Build history of the part. All positions in model axes, mm. Face numbers are marked on the shaded views. A direction names the side the tool comes from. Coordinates: 2 decimals unless noted, no trailing zeros. Loops run counter-clockwise (first coordinate to the right, second up) from the corner with the lowest first, then second, coordinate; pieces in that order, holes last.
Item 1: Cut at A-A (y = 2.5). Count the separate pieces of the cut face and the enclosed holes in it, and give its area (3 significant figures).
Item 2: Cut at B-B (x = 2.5). List the corners of the cut face in (y, z) (3 decimals).
Item 3: Mould opens along X. For the marked faces 1, 2, 3 and 4 say: released by +X, released by -X, zero draft, split by the parting line, or undercut.
Item 4: 3-axis set-ups, long thin cutter, end or side, ignore diameter. For the marked faces 5, 6 and 7: which of +Z, -Z, +X, -X, +Y, -Y reach the whole face in a straight line?
Item 5: Drill centre lines: line 1 along X through (y, z) = (6.25, -0.9); line 2 along X through (y, z) = (6.5, 0.3) (3 decimals); line 3 along X through (y, z) = (5.5, -0.1). Where is each one in solid material? Low to high.
Item 6: Flat gauge pins, fed straight in: pin 1 (2 mm diameter, centred on x = 3.5, z = 2.5, fed in from +Y); pin 2 (0.8 mm diameter, centred on x = -3, z = -2, fed in from -Y). Where does each tip first touch, or does it go through?
Item 7: Cut at D-D (y = 4.75). List the corners of the cut face in (x, z), and give its area (3 significant figures).
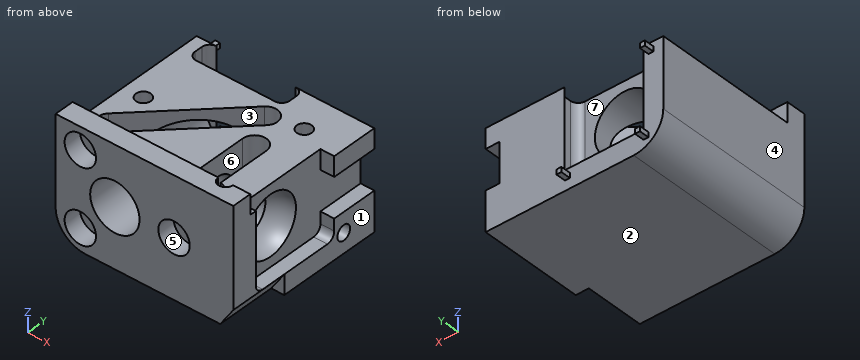
from build123d import *

# Parameters (mm, degrees)
SKETCH1_W                       = 9
SKETCH1_H                       = 6
MAIN_BODY_EXT_DEPTH             = 8.3
EMISSION_PATH_EXT_DEPTH         = 9
SKETCH3_R                       = 1.25
EMISSION_AND_GRIN_CUT_DEPTH     = 19.125672401
SKETCH4_R                       = 1
DRUM_LENS_CUT_DEPTH             = 7
SKETCH5_W                       = 9
SKETCH5_H                       = 7.3
FILTERSET_CUT1_DEPTH            = 1
FILTERSET_CUT2_DEPTH            = 4
SKETCH10_R                      = 2.5
EMISSION_LENS_CUT_DEPTH         = 8.5
SKETCH15_R                      = 0.795
MAGNETS_CUT_DEPTH               = 0.9
SCREW_HOLES_CUT_DEPTH           = 19.561788707
SCREW_HOLES_CUT_DEPTH_BACK      = 3
SKETCH18_R                      = 0.375
EXTERNAL_FILLET_1_R             = 1.5
CUT_EXTRUDE8_DEPTH              = 12.545128843
CUT_EXTRUDE8_DEPTH_BACK         = 4
SKETCH28_R                      = 1.5
CUT_EXTRUDE9_DEPTH              = 3
CUT_EXTRUDE10_DEPTH             = 0.7
SKETCH29_R                      = 0.375
CUT_EXTRUDE11_DEPTH             = 2.5
SKETCH32_W                      = 2
SKETCH32_H                      = 2.36
CUT_EXTRUDE14_DEPTH             = 0.7
CUT_EXTRUDE16_DEPTH             = 9
CUT_EXTRUDE17_REACH             = 12.329
SKETCH37_R                      = 2
CUT_EXTRUDE18_START             = -9
CUT_EXTRUDE18_DEPTH             = 9
CUT_EXTRUDE19_REACH             = 20.126
SKETCH39_W                      = 5.765434423
SKETCH39_H                      = 9
CUT_EXTRUDE19_DIRECTION_2_REACH = 20.126
SKETCH40_W                      = 0.25
SKETCH40_H                      = 0.25
BOSS_EXTRUDE1_DEPTH             = 0.5


with BuildPart() as part:
    # Sketch1 → Main Body Ext (new body)
    with BuildSketch(Plane(origin=(0, 0, 0), x_dir=(1, 0, 0), z_dir=(0, 1, 0))):
        Rectangle(SKETCH1_W, SKETCH1_H)
    extrude(amount=MAIN_BODY_EXT_DEPTH)

    # Sketch8 → Emission Path Ext (add)
    with BuildSketch(Plane(origin=(0, 8.3, 0), x_dir=(1, 0, 0), z_dir=(0, 1, 0))):
        Polygon((0.25, 3), (1.5, 1.75), (1.5, -3), (-4.5, -3), (-4.5, 3), align=None)
    extrude(amount=EMISSION_PATH_EXT_DEPTH)

    # Sketch3 → Emission and Grin Cut (cut, through all)
    with BuildSketch(Plane.XZ):
        with Locations(Location((-1.5, 0, 0), (0, 0, 270))):
            Circle(SKETCH3_R)
    extrude(amount=-EMISSION_AND_GRIN_CUT_DEPTH, mode=Mode.SUBTRACT)

    # Sketch4 → Drum Lens Cut (cut)
    with BuildSketch(Plane(origin=(4.5, 0, 0), x_dir=(0, 0, -1), z_dir=(1, 0, 0))):
        with Locations((0, 3)):
            Circle(SKETCH4_R)
    extrude(amount=-DRUM_LENS_CUT_DEPTH, mode=Mode.SUBTRACT)

    # Sketch5 → FilterSet Cut1 (cut)
    with BuildSketch(Plane.XY.offset(3)):
        with Locations((0, 4.65)):
            Rectangle(SKETCH5_W, SKETCH5_H)
    extrude(amount=-FILTERSET_CUT1_DEPTH, mode=Mode.SUBTRACT)

    # Sketch6 → FilterSet Cut2 (cut)
    with BuildSketch(Plane.XY.offset(2)):
        with BuildLine():
            Line((2.3, 4.5), (2.3, 1.8))
            ThreePointArc((2.3, 1.8), (2.7, 1.4), (2.3, 1))
            Line((2.3, 1), (1.1, 1))
            ThreePointArc((1.1, 1), (0.7, 1.4), (1.1, 1.8))
            Line((1.1, 1.8), (1.1, 4.5))
            ThreePointArc((1.1, 4.5), (1.7, 5.1), (2.3, 4.5))
        make_face()
        with BuildLine():
            Line((-3.9, 7.9), (-3.9, 7.5))
            ThreePointArc((-3.9, 7.5), (-3.782842712, 7.217157288), (-3.5, 7.1))
            Line((-3.5, 7.1), (0.5, 7.1))
            ThreePointArc((0.5, 7.1), (0.782842712, 7.217157288), (0.9, 7.5))
            Line((0.9, 7.5), (0.9, 7.9))
            ThreePointArc((0.9, 7.9), (0.782842712, 8.182842712), (0.5, 8.3))
            Line((0.5, 8.3), (-3.5, 8.3))
            ThreePointArc((-3.5, 8.3), (-3.782842712, 8.182842712), (-3.9, 7.9))
        make_face()
        with BuildLine():
            Line((0.39411255, 6.591168825), (-3.848528137, 2.348528137))
            ThreePointArc((-3.848528137, 2.348528137), (-3.848528137, 1.5), (-3, 1.5))
            Line((-3, 1.5), (1.242640687, 5.742640687))
            ThreePointArc((1.242640687, 5.742640687), (1.242640687, 6.591168825), (0.39411255, 6.591168825))
        make_face()
    extrude(amount=-FILTERSET_CUT2_DEPTH, mode=Mode.SUBTRACT)

    # Sketch10 → Emission Lens Cut (cut)
    with BuildSketch(Plane(origin=(0, 17.3, 0), x_dir=(1, 0, 0), z_dir=(0, 1, 0))):
        with Locations(Location((-1.5, 0, 0), (0, 0, 270))):
            Circle(SKETCH10_R)
    extrude(amount=-EMISSION_LENS_CUT_DEPTH, mode=Mode.SUBTRACT)

    # Sketch15 → Magnets Cut (cut)
    with BuildSketch(Plane.XZ):
        with Locations(Location((-3.25, -1.875, 0), (0, 0, 270))):
            Circle(SKETCH15_R)
        with Locations(Location((-3.25, 1.875, 0), (0, 0, 270))):
            Circle(SKETCH15_R)
        with Locations(Location((1.5, 0, 0), (0, 0, 270))):
            Circle(SKETCH15_R)
    extrude(amount=-MAGNETS_CUT_DEPTH, mode=Mode.SUBTRACT)

    # Sketch18 → Screw Holes Cut (cut, two sides: drawn at the far end of the back side and taken through both)
    with BuildSketch(Plane.XY.offset(2).offset(-SCREW_HOLES_CUT_DEPTH_BACK)):
        with Locations(Location((-3.5, 4, 0), (0, 0, 180))):
            Circle(SKETCH18_R)
        with Locations(Location((2.5, 6.5, 0), (0, 0, 180))):
            Circle(SKETCH18_R)
        with Locations((3.25, 1)):
            Circle(SKETCH18_R)
    extrude(amount=SCREW_HOLES_CUT_DEPTH + SCREW_HOLES_CUT_DEPTH_BACK, mode=Mode.SUBTRACT)

    # External Fillet 1
    # the kernel refuses this fillet: 1.5 mm, written as the material it takes off along each edge
    with BuildSketch(Plane(origin=(-4.5, -3.75, -3), x_dir=(1, 0, 0), z_dir=(0, 1, 0))) as external_fillet_1_piece_1:
        with BuildLine():
            CenterArc((EXTERNAL_FILLET_1_R, -EXTERNAL_FILLET_1_R), EXTERNAL_FILLET_1_R, 90, 90)
            Line((0, -EXTERNAL_FILLET_1_R), (0, 0))
            Line((0, 0), (EXTERNAL_FILLET_1_R, 0))
        make_face()
    extrude(amount=24.8, mode=Mode.SUBTRACT)
    with BuildSketch(Plane(origin=(1.5, 8.3, 3), x_dir=(0, 0, -1), z_dir=(0, 1, 0))) as external_fillet_1_piece_2:
        with BuildLine():
            CenterArc((EXTERNAL_FILLET_1_R, EXTERNAL_FILLET_1_R), EXTERNAL_FILLET_1_R, 180, 90)
            Line((0, EXTERNAL_FILLET_1_R), (0, 0))
            Line((0, 0), (EXTERNAL_FILLET_1_R, 0))
        make_face()
    extrude(amount=12.75, mode=Mode.SUBTRACT)

    # Sketch28 → Cut-Extrude8 (cut, two sides: drawn at the far end of the back side and taken through both)
    with BuildSketch(Plane(origin=(0, 7.1, 0), x_dir=(1, 0, 0), z_dir=(0, 1, 0)).offset(-CUT_EXTRUDE8_DEPTH_BACK)):
        with Locations(Location((-1.5, 0, 0), (0, 0, 180))):
            Circle(SKETCH28_R)
    extrude(amount=CUT_EXTRUDE8_DEPTH + CUT_EXTRUDE8_DEPTH_BACK, mode=Mode.SUBTRACT)

    # Sketch14 → Cut-Extrude9 (cut)
    with BuildSketch(Plane.XZ):
        Polygon((4.5, -3), (4.5, -2.006698359), (3.837798906, -3), align=None)
    extrude(amount=-CUT_EXTRUDE9_DEPTH, mode=Mode.SUBTRACT)

    # Sketch12 → Cut-Extrude10 (cut)
    with BuildSketch(Plane(origin=(4.5, 0, 0), x_dir=(0, 0, -1), z_dir=(1, 0, 0))):
        with BuildLine():
            Line((1.6, 5.94), (-1.6, 5.94))
            Line((-1.6, 5.94), (-2, 5.94))
            Line((-2, 5.94), (-2, 1.33))
            Line((-2, 1.33), (1.6, 1.33))
            ThreePointArc((1.6, 1.33), (1.882842712, 1.447157288), (2, 1.73))
            Line((2, 1.73), (2, 5.54))
            ThreePointArc((2, 5.54), (1.882842712, 5.822842712), (1.6, 5.94))
        make_face()
    extrude(amount=-CUT_EXTRUDE10_DEPTH, mode=Mode.SUBTRACT)

    # Sketch29 → Cut-Extrude11 (cut)
    with BuildSketch(Plane(origin=(4.5, 0, 0), x_dir=(0, 0, -1), z_dir=(1, 0, 0))):
        with Locations((2, 6.5)):
            Circle(SKETCH29_R)
    extrude(amount=-CUT_EXTRUDE11_DEPTH, mode=Mode.SUBTRACT)

    # Sketch32 → Cut-Extrude14 (cut)
    with BuildSketch(Plane(origin=(4.5, 0, 0), x_dir=(0, 0, -1), z_dir=(1, 0, 0))):
        with Locations((0, 7.12)):
            Rectangle(SKETCH32_W, SKETCH32_H)
    extrude(amount=-CUT_EXTRUDE14_DEPTH, mode=Mode.SUBTRACT)

    # Sketch33 → Cut-Revolve1 (revolve, cut)
    with BuildSketch(Plane.XY, mode=Mode.PRIVATE) as cut_revolve1_sk:
        with BuildLine():
            Line((3.8, 3), (2.3, 3))
            ThreePointArc((2.3, 3), (2.739339828, 4.060660172), (3.8, 4.5))
            Line((3.8, 4.5), (3.8, 3))
        make_face()
    revolve(cut_revolve1_sk.sketch.rotate(Axis((3.8, 3, 0), (-1, 0, 0)), 90), axis=Axis((3.8, 3, 0), (-1, 0, 0)), mode=Mode.SUBTRACT)

    # Sketch36 → Cut-Extrude16 (cut)
    with BuildSketch(Plane(origin=(0, 17.3, 0), x_dir=(1, 0, 0), z_dir=(0, 1, 0))):
        with BuildLine():
            Line((-4.5, -1.5), (-4.5, -3))
            Line((-4.5, -3), (-3, -3))
            ThreePointArc((-3, -3), (-4.060660172, -2.560660172), (-4.5, -1.5))
        make_face()
    extrude(amount=-CUT_EXTRUDE16_DEPTH, mode=Mode.SUBTRACT)

    # Sketch37 → Cut-Extrude17 (cut, up to next)
    with BuildSketch(Plane(origin=(0, 8.8, 0), x_dir=(1, 0, 0), z_dir=(0, 1, 0)), mode=Mode.PRIVATE) as cut_extrude17_sk1:
        with Locations(Location((-1.5, 0, 0), (0, 0, 180))):
            Circle(SKETCH37_R)
    cut_extrude17_tool1 = extrude(cut_extrude17_sk1.sketch, amount=-CUT_EXTRUDE17_REACH, mode=Mode.PRIVATE) & part.part
    add(cut_extrude17_tool1.solids().sort_by_distance((-1.5, 8.8, 0))[0], mode=Mode.SUBTRACT)

    # Sketch38 → Cut-Extrude18 (cut)
    with BuildSketch(Plane(origin=(0, 17.3, 0), x_dir=(1, 0, 0), z_dir=(0, 1, 0)).offset(CUT_EXTRUDE18_START)):
        with BuildLine():
            Line((-3, 3), (0.25, 3))
            Line((0.25, 3), (1.5, 1.75))
            Line((1.5, 1.75), (1.5, -1.5))
            ThreePointArc((1.5, -1.5), (1.060660172, -2.560660172), (0, -3))
            Line((0, -3), (-3, -3))
            ThreePointArc((-3, -3), (-4.060660172, -2.560660172), (-4.5, -1.5))
            Line((-4.5, -1.5), (-4.5, 1.5))
            ThreePointArc((-4.5, 1.5), (-4.060660172, 2.560660172), (-3, 3))
        make_face()
        with BuildLine():
            Line((-4.375, -1.5), (-4.375, 1.5))
            ThreePointArc((-4.375, 1.5), (-3.940482173, 2.440482173), (-3, 2.875))
            Line((-3, 2.875), (0.25, 2.875))
            Line((0.25, 2.875), (1.375, 1.75))
            Line((1.375, 1.75), (1.375, -1.5))
            ThreePointArc((1.375, -1.5), (0.972271824, -2.472271824), (0, -2.875))
            Line((0, -2.875), (-3, -2.875))
            ThreePointArc((-3, -2.875), (-3.972271824, -2.472271824), (-4.375, -1.5))
        make_face(mode=Mode.SUBTRACT)
    extrude(amount=CUT_EXTRUDE18_DEPTH, mode=Mode.SUBTRACT)

    # Cut-Extrude19: up to this face of the body (flat: up to its plane)
    cut_extrude19_end = Plane(part.part.faces().sort_by_distance((-1.375, 12.8, -2.875))[0])
    # Sketch39 → Cut-Extrude19 (cut, up to the picked face)
    with BuildSketch(Plane.XY, mode=Mode.PRIVATE) as cut_extrude19_sk1:
        with Locations((-1.507717212, 12.8)):
            Rectangle(SKETCH39_W, SKETCH39_H)
    cut_extrude19_tool1 = split(extrude(cut_extrude19_sk1.sketch, amount=-CUT_EXTRUDE19_REACH, mode=Mode.PRIVATE), bisect_by=cut_extrude19_end, keep=Keep.BOTH, mode=Mode.PRIVATE)
    add(cut_extrude19_tool1.solids().sort_by(Axis((-1.507717, 12.8, 0), (0, 0, -1)))[0], mode=Mode.SUBTRACT)

    # Cut-Extrude19 direction 2: up to this face of the body (flat: up to its plane)
    cut_extrude19_direction_2_end = Plane(part.part.faces().sort_by_distance((-1.5, 12.8, 2.875))[0])
    # Sketch39 → Cut-Extrude19 direction 2 (cut, up to the picked face)
    with BuildSketch(Plane.XY, mode=Mode.PRIVATE) as cut_extrude19_direction_2_sk1:
        with Locations((-1.507717212, 12.8)):
            Rectangle(SKETCH39_W, SKETCH39_H)
    cut_extrude19_direction_2_tool1 = split(extrude(cut_extrude19_direction_2_sk1.sketch, amount=CUT_EXTRUDE19_DIRECTION_2_REACH, mode=Mode.PRIVATE), bisect_by=cut_extrude19_direction_2_end, keep=Keep.BOTH, mode=Mode.PRIVATE)
    add(cut_extrude19_direction_2_tool1.solids().sort_by(Axis((-1.507717, 12.8, 0), (0, 0, 1)))[0], mode=Mode.SUBTRACT)

    # Sketch40 → Boss-Extrude1 (add)
    with BuildSketch(Plane(origin=(0, 8.3, 0), x_dir=(1, 0, 0), z_dir=(0, 1, 0))):
        with Locations((-3.625, 2.375)):
            Rectangle(SKETCH40_W, SKETCH40_H)
        with Locations((0.353060916, 2.375)):
            Rectangle(SKETCH40_W, SKETCH40_H)
        with Locations((-3.875, -1.625)):
            Rectangle(SKETCH40_W, SKETCH40_H)
    extrude(amount=BOSS_EXTRUDE1_DEPTH)


solid = part.part
Filled sheet:
1. separate pieces: 3
1. enclosed holes: 0
1. area: 20.1 mm2
2. outline: (0, -3) - (8.3, -3) - (8.3, 2) - (6.875, 2) - (6.875, -1) - (6.125, -1) - (6.125, 2) - (1.746, 2) - (1.746, -2) - (1.054, -2) - (1.054, 2) - (1, 2) - (1, 3) - (0, 3) - close; hole circle Ø2 at (3, 0); hole circle Ø0.75 at (6.5, -2)
3. face 1: released by +X
3. face 2: zero draft
3. face 3: undercut
3. face 4: released by -X
4. face 5: -Y
4. face 6: +Z
4. face 7: +Z, +Y
5. line 1: x = -4.5 to -2.7, -0.3 to 0.05, 1.41 to 2.22, 2.78 to 3.8
5. line 2: x = -4.5 to -2.97, -0.03 to 0.303, 1.317 to 2.125, 2.875 to 3.8
5. line 3: x = -4.5 to -3, 1 to 3.8
6. pin 1: stops at y = 8.3
6. pin 2: stops at y = 0.9
7. outline: (-4.5, -1.5) arc R1.5 ccw to (-3, -3) - (4.5, -3) - (4.5, -2) - (3.8, -2) - (3.8, 2) - (2.25, 2) - (2.25, -2) - (1.15, -2) - (1.15, 2) - (0.25, 2) - (0.25, -2) - (-1.45, -2) - (-1.45, -1.5) arc R1.5 cw (long way) to (-1.45, 1.5) - (-1.45, 2) - (-4.5, 2) - close
7. area: 26.9 mm2
